from build123d import *

# Parameters (mm, degrees)
SKETCH1_W           = 15.494
SKETCH1_H           = 12.7
SKETCH1_R           = 3.2639
SKETCH1_W_2         = 22.352
BOSS_EXTRUDE3_DEPTH = 3.81
SKETCH3_W           = 20.828
SKETCH3_H           = 12.7
BOSS_EXTRUDE4_DEPTH = 15.24
CUT_EXTRUDE2_REACH  = 14.7


with BuildPart() as part:
    # Sketch1 → Boss-Extrude3 (new body)
    with BuildSketch(Plane(origin=(0, 0, 0), x_dir=(1, 0, 0), z_dir=(0, 1, 0))):
        with Locations((-27.634045528, -3.236090754)):
            Rectangle(SKETCH1_W, SKETCH1_H)
        with Locations((-27.507045528, -3.236090754)):
            Circle(SKETCH1_R, mode=Mode.SUBTRACT)
        with Locations((-8.711045528, -3.236090754)):
            Rectangle(SKETCH1_W_2, SKETCH1_H)
        with Locations((10.211954472, -3.236090754)):
            Rectangle(SKETCH1_W, SKETCH1_H)
        with Locations((10.084954472, -3.236090754)):
            Circle(SKETCH1_R, mode=Mode.SUBTRACT)
    extrude(amount=BOSS_EXTRUDE3_DEPTH)

    # Sketch3 → Boss-Extrude4 (add)
    with BuildSketch(Plane(origin=(0, 3.81, 0), x_dir=(1, 0, 0), z_dir=(0, 1, 0))):
        with Locations((-8.711045528, -3.236090754)):
            Rectangle(SKETCH3_W, SKETCH3_H)
    extrude(amount=BOSS_EXTRUDE4_DEPTH)

    # Sketch4 → Cut-Extrude2 (cut, up to next)
    with BuildSketch(Plane.XY.offset(9.586090754), mode=Mode.PRIVATE) as cut_extrude2_sk1:
        Polygon((-8.262769146, 18.127348419), (-14.612769146, 14.461174209), (-14.612769146, 7.128825791), (-8.262769146, 3.462651581), (-1.912769146, 7.128825791), (-1.912769146, 14.461174209), align=None)
    cut_extrude2_tool1 = extrude(cut_extrude2_sk1.sketch, amount=-CUT_EXTRUDE2_REACH, mode=Mode.PRIVATE) & part.part
    add(cut_extrude2_tool1.solids().sort_by_distance((-8.262769, 10.795, 9.586091))[0], mode=Mode.SUBTRACT)


solid = part.part
Input: part model. Units: mm. Frame: model coordinates. A direction names the side the tool comes from. Coordinates: 2 decimals unless noted, no trailing zeros. Loops run counter-clockwise (first coordinate to the right, second up) from the corner with the lowest first, then second, coordinate; pieces in that order, holes last. Notation, with made-up numbers: (-20.5, -3.5) -> (-16.5, -3.5) arc R18 cw to (-16.5, 22.5) -> close; hole circle Ø5 at (-7, 61). An arc over 180 degrees is marked (long way). Write item = value, one per line. Start each with the question number.
Item 1: Cut plane C-C, the plane y = 9.5. Return loops of the section in (x, z), plus the area to 3 significant figures.
Item 2: Cut plane D-D, the plane x = -26.5. Return loops of the section in (y, z).
Item 3: Cut plane B-B, the plane z = -1.75. Return loops of the section in (x, y).
Item 4: Reachability of faces 1 (the face through (-11.48, 5.32, 3.32)), 2 (the face through (-9, 0, 3)), 3 (the face through (-19.125, 11, 3)), 4 (the face through (1.703, 11, 3)) from +Z, -Z, +X, -X, +Y, -Y: full face, straight path, thin tool, end or side. Return the list, or none.
Item 5: Material intervals for line 1 (X direction, y = 10, z = 0.5); line 2 (Y direction, x = -33, z = -0.75); line 3 (X direction, y = 6.75, z = 6.5), sorted ascending.
Item 6: Mould query, pull axis Z, two halves, no side actions, for faces 5 (the face through (6.824, 1.878, 3.093)), 6 (the face through (-9, 3, -3.114)), 7 (the face through (-28.215, 1.878, 6.422)), 8 (the face through (17.959, 2, 3)). Classes: pulls with the +Z half, pulls with the -Z half, needs draft (parallel to the pull), parting line crosses it, or undercut.
Item 7: First-contact query: P1, Ø5, axis at y = 14.5, z = 7.5, coming from the +X side; P2, Ø4, axis at y = 14, z = 2.5, coming from the -X side; P3, Ø2, axis at x = -28, z = 7, coming from the +Y side; P4, Ø4, axis at x = -27.51, z = 3.24, coming from the +Y side. Flat tips, straight axial feed; report the tip coordinate or a pass-through.
Item 8: Cut plane A-A, the plane z = 5.5. Return loops of the section in (x, y), plus the area to 3 significant figures.
Ans:
q1.outline = (-19.13, -3.11) -> (-14.61, -3.11) -> (-14.61, 9.59) -> (-19.13, 9.59) -> close; (-1.91, -3.11) -> (1.7, -3.11) -> (1.7, 9.59) -> (-1.91, 9.59) -> close
q1.area = 103 mm²
q2.outline = (0, -3.11) -> (3.81, -3.11) -> (3.81, 0.13) -> (0, 0.13) -> close; (0, 6.34) -> (3.81, 6.34) -> (3.81, 9.59) -> (0, 9.59) -> close
q3.outline = (-35.38, 0) -> (17.96, 0) -> (17.96, 3.81) -> (1.7, 3.81) -> (1.7, 19.05) -> (-19.13, 19.05) -> (-19.13, 3.81) -> (-35.38, 3.81) -> close; hole (-14.61, 7.13) -> (-8.26, 3.46) -> (-1.91, 7.13) -> (-1.91, 14.46) -> (-8.26, 18.13) -> (-14.61, 14.46) -> close
q4.face_1 = +Z, -Z
q4.face_2 = +Z, -Z, +X, -X, -Y
q4.face_3 = +Z, -Z, -X, +Y
q4.face_4 = +Z, -Z, +X, +Y
q5.line_1 = -19.13 to -14.61, -1.91 to 1.7
q5.line_2 = 0 to 3.81
q5.line_3 = -19.13 to -13.96, -2.57 to 1.7
q6.face_5 = undercut
q6.face_6 = pulls with the -Z half
q6.face_7 = undercut
q6.face_8 = needs draft
q7.P1 = 1.7
q7.P2 = -19.13
q7.P3 = 3.81
q7.P4 = through
q8.outline = (-35.38, 0) -> (-29.86, 0) -> (-29.86, 3.81) -> (-35.38, 3.81) -> close; (-25.16, 0) -> (7.73, 0) -> (7.73, 3.81) -> (1.7, 3.81) -> (1.7, 19.05) -> (-19.13, 19.05) -> (-19.13, 3.81) -> (-25.16, 3.81) -> close; (12.44, 0) -> (17.96, 0) -> (17.96, 3.81) -> (12.44, 3.81) -> close; hole (-14.61, 7.13) -> (-8.26, 3.46) -> (-1.91, 7.13) -> (-1.91, 14.46) -> (-8.26, 18.13) -> (-14.61, 14.46) -> close
q8.area = 345 mm²
